Geometry check sheet. Reference: the model listing, model coordinates, mm. Round coordinates to 2 decimals unless told otherwise and drop trailing zeros. Order: outer loops, then holes, each group sorted by start corner. A loop starts at its lowest first (then second) coordinate and runs counter-clockwise, first axis right, second up. Notation, with made-up numbers: (77, -17.75) -> (97, -17.75) arc R21 cw to (97, -11.75) -> close; hole circle Ø7 at (48, 84). An arc over 180 degrees is marked (long way). Use a Markdown table: item, result. Add a question column.
Item 1: Sectioned sample at C-C, the plane z = -47. State how many separate pieces and enclosed holes the cut face has, and give its area (3 significant figures).
Item 2: Sectioned sample at A-A, the plane y = 1.15. Record the cut outline in (x, z), and give its area (3 significant figures).
Item 3: Material ranges on probe 1 along X at (y, z) = (3, -41); probe 2 along Z at (x, y) = (-34, 4.5); probe 3 along Z at (x, y) = (-179, 4.55), recorded low to high. Write a range as [from, to].
Item 4: Sectioned sample at B-B, the plane x = -60. Record the cut outline in (y, z), and give its area (4 significant figures).
Item 5: Mould release check, pull along X, two halves, no side actions. Record for faces 1 (the cylindrical face through (-240.16, 2.54, -42.5)), 2 (the flat face through (-157, 2, 0)), 3 (the flat face through (0, 2, -25)): pulls with the +X half, pulls with the -X half, needs draft (parallel to the pull), parting line crosses it, or undercut.
from build123d import *

# Parameters (mm, degrees)
SKETCH1_W           = 300
SKETCH1_H           = 50
BOSS_EXTRUDE1_DEPTH = 5
SKETCH2_R           = 7.5
CUT_EXTRUDE1_DEPTH  = 5
LPATTERN1_COUNT     = 9
LPATTERN1_PITCH     = 30
FILLET2_R           = 10


with BuildPart() as part:
    # Sketch1 → Boss-Extrude1 (new body)
    with BuildSketch(Plane(origin=(0, 0, 0), x_dir=(1, 0, 0), z_dir=(0, 1, 0))):
        with Locations((-150, 25)):
            Rectangle(SKETCH1_W, SKETCH1_H)
    extrude(amount=BOSS_EXTRUDE1_DEPTH)

    # Sketch2 → Cut-Extrude1 (cut)
    with BuildSketch(Plane(origin=(0, 5, 0), x_dir=(1, 0, 0), z_dir=(0, 1, 0))):
        with Locations((-270, 50)):
            Circle(SKETCH2_R)
    cut_extrude1 = extrude(amount=-CUT_EXTRUDE1_DEPTH, mode=Mode.SUBTRACT)

    # LPattern1: Cut-Extrude1 ×9
    with Locations(*[(i * LPATTERN1_PITCH, 0, 0) for i in range(1, LPATTERN1_COUNT)]):
        add(cut_extrude1, mode=Mode.SUBTRACT)

    # Fillet2
    fillet2_edges = [part.edges().sort_by_distance(p)[0] for p in [
        (0, 2.5, 0),
        (0, 2.5, -50),
    ]]
    fillet(fillet2_edges, radius=FILLET2_R)


solid = part.part
Found:
| question | item | result |
|---|---|---|
| 1 | separate pieces | 10 |
| 1 | enclosed holes | 0 |
| 1 | area | 867 mm2 |
| 2 | outline | (-300, -50) -> (-277.5, -50) arc R7.5 cw to (-262.5, -50) -> (-247.5, -50) arc R7.5 cw to (-232.5, -50) -> (-217.5, -50) arc R7.5 cw to (-202.5, -50) -> (-187.5, -50) arc R7.5 cw to (-172.5, -50) -> (-157.5, -50) arc R7.5 cw to (-142.5, -50) -> (-127.5, -50) arc R7.5 cw to (-112.5, -50) -> (-97.5, -50) arc R7.5 cw to (-82.5, -50) -> (-67.5, -50) arc R7.5 cw to (-52.5, -50) -> (-37.5, -50) arc R7.5 cw to (-22.5, -50) -> (-10, -50) arc R10 ccw to (0, -40) -> (0, -10) arc R10 ccw to (-10, 0) -> (-300, 0) -> close |
| 2 | area | 14,200 mm2 |
| 3 | probe 1 | x = [-300, -0.05] |
| 3 | probe 2 | z = [-43.66, 0] |
| 3 | probe 3 | z = [-42.57, 0] |
| 4 | outline | (0, -42.5) -> (5, -42.5) -> (5, 0) -> (0, 0) -> close |
| 4 | area | 212.5 mm2 |
| 5 | face 1 | undercut |
| 5 | face 2 | needs draft |
| 5 | face 3 | pulls with the +X half |
